Design review of the part shown in the three views and the two pictorial views. Dimensions are in mm from the part's minimum x, y and z. Coordinates: 2 decimals unless noted, no trailing zeros. Loops run counter-clockwise (first coordinate to the right, second up) from the corner with the lowest first, then second, coordinate; pieces in that order, holes last. Notation, with made-up numbers: (51, 38.25) - (86, 38.25) arc R25 ccw to (86, 73.25) - close; hole circle Ø2 at (-4, -9.75). An arc over 180 degrees is marked (long way). One line per item, written item: value. Start each with the question number.
1. Take a section at B-B, the plane y = 2.05. State the section outline as (x, z) points.
2. To check wall thickness, follow line 1 (Z direction, x = 15.5, y = 1.8); line 2 (X direction, y = 1.25, z = 26). State the ranges of each line that lie inside material, in increasing order. Write a range as from..to.
3. Take a section at A-A, the plane x = 17.5. State the section outline as (y, z) points, and give its area (3 significant figures).
4. Insertion check: pin 1 (2.5 mm diameter, centred on y = 2.5, z = 8, fed in from +X); pin 2 (2.5 mm diameter, centred on x = 18, y = 2.5, fed in from +Z). Each pin has a flat end and moves straight along its axis. Give the tip position at first contact, or say it passes through.
5. Take a section at C-C, the plane z = 75. State the section outline as (x, y) points, and give its area (3 significant figures).
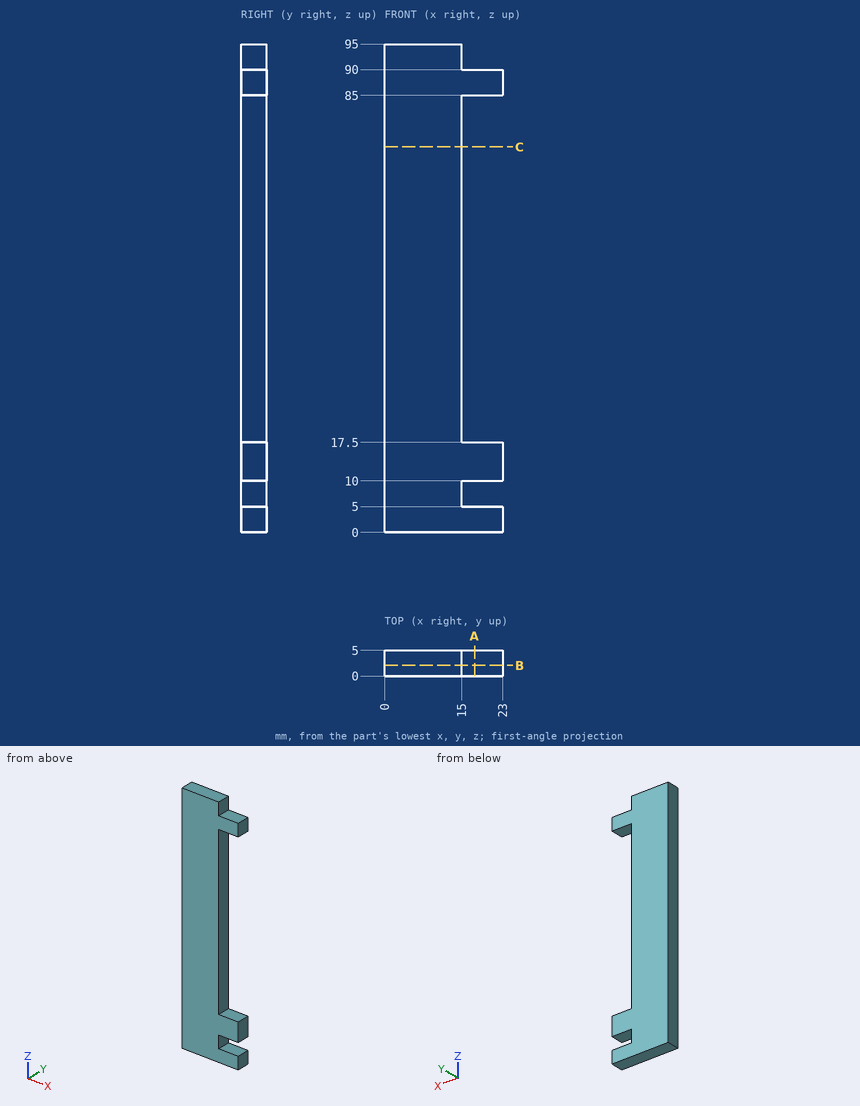
Solutions:
1. outline: (0, 0) - (23, 0) - (23, 5) - (15, 5) - (15, 10) - (23, 10) - (23, 17.5) - (15, 17.5) - (15, 85) - (23, 85) - (23, 90) - (15, 90) - (15, 95) - (0, 95) - close
2. line 1: 0..5, 10..17.5, 85..90
2. line 2: 0..15
3. outline: (0, 0) - (5, 0) - (5, 5) - (0, 5) - close; (0, 10) - (5, 10) - (5, 17.5) - (0, 17.5) - close; (0, 85) - (5, 85) - (5, 90) - (0, 90) - close
3. area: 87.5 mm2
4. pin 1: x = 15
4. pin 2: z = 90
5. outline: (0, 0) - (15, 0) - (15, 5) - (0, 5) - close
5. area: 75.0 mm2
